from build123d import *

# Parameters (mm, degrees)
SKETCH2_R            = 15.875
BOSS_EXTRUDE1_DEPTH  = 25.4
SKETCH4_R            = 19.05
BOSS_EXTRUDE2_DEPTH  = 25.4
SKETCH5_R            = 22.225
BOSS_EXTRUDE3_DEPTH  = 3.175
SKETCH6_R            = 19.05
BOSS_EXTRUDE4_DEPTH  = 3.175
SKETCH7_R            = 22.225
BOSS_EXTRUDE5_DEPTH  = 43.5102
SKETCH8_R            = 25.4
BOSS_EXTRUDE6_DEPTH  = 77.1398
CUT_EXTRUDE1_DEPTH   = 3.175
SKETCH10_R           = 12.7
BOSS_EXTRUDE7_DEPTH  = 3.175
SKETCH11_R           = 15.875
BOSS_EXTRUDE8_DEPTH  = 3.175
SKETCH12_R           = 12.7
BOSS_EXTRUDE9_DEPTH  = 3.175
SKETCH13_R           = 15.875
BOSS_EXTRUDE10_DEPTH = 3.175


with BuildPart() as part:
    # Sketch2 → Boss-Extrude1 (new body)
    with BuildSketch(Plane.XY):
        Circle(SKETCH2_R)
    extrude(amount=BOSS_EXTRUDE1_DEPTH)

    # Sketch4 → Boss-Extrude2 (add)
    with BuildSketch(Plane.XY.offset(25.4)):
        Circle(SKETCH4_R)
    extrude(amount=BOSS_EXTRUDE2_DEPTH)

    # Sketch5 → Boss-Extrude3 (add)
    with BuildSketch(Plane.XY.offset(50.8)):
        Circle(SKETCH5_R)
    extrude(amount=BOSS_EXTRUDE3_DEPTH)

    # Sketch6 → Boss-Extrude4 (add)
    with BuildSketch(Plane.XY.offset(53.975)):
        Circle(SKETCH6_R)
    extrude(amount=BOSS_EXTRUDE4_DEPTH)

    # Sketch7 → Boss-Extrude5 (add)
    with BuildSketch(Plane.XY.offset(57.15)):
        Circle(SKETCH7_R)
    extrude(amount=BOSS_EXTRUDE5_DEPTH)

    # Sketch8 → Boss-Extrude6 (add)
    with BuildSketch(Plane.XY.offset(100.6602)):
        Circle(SKETCH8_R)
    extrude(amount=BOSS_EXTRUDE6_DEPTH)

    # Sketch9 → Cut-Extrude1 (cut)
    with BuildSketch(Plane(origin=(0, -22.225, 0), x_dir=(-1, 0, 0), z_dir=(0, -1, 0))):
        with BuildLine():
            Line((3.175, -69.3801), (3.175, -88.4301))
            ThreePointArc((3.175, -88.4301), (0, -91.6051), (-3.175, -88.4301))
            Line((-3.175, -88.4301), (-3.175, -69.3801))
            ThreePointArc((-3.175, -69.3801), (0, -66.2051), (3.175, -69.3801))
        make_face()
    extrude(amount=-CUT_EXTRUDE1_DEPTH, mode=Mode.SUBTRACT)

    # Mirror1: part across plane


with BuildPart() as part_1:
    add(part.part)
    add(part.part.mirror(Plane.XY.offset(177.8)))

    # Sketch10 → Boss-Extrude7 (add)
    with BuildSketch(Plane(origin=(0, 0, 0), x_dir=(-1, 0, 0), z_dir=(0, 0, -1))):
        Circle(SKETCH10_R)
    extrude(amount=BOSS_EXTRUDE7_DEPTH)

    # Sketch11 → Boss-Extrude8 (add)
    with BuildSketch(Plane(origin=(0, 0, -3.175), x_dir=(-1, 0, 0), z_dir=(0, 0, -1))):
        Circle(SKETCH11_R)
    extrude(amount=BOSS_EXTRUDE8_DEPTH)

    # Sketch12 → Boss-Extrude9 (add)
    with BuildSketch(Plane.XY.offset(355.6)):
        Circle(SKETCH12_R)
    extrude(amount=BOSS_EXTRUDE9_DEPTH)

    # Sketch13 → Boss-Extrude10 (add)
    with BuildSketch(Plane.XY.offset(358.775)):
        Circle(SKETCH13_R)
    extrude(amount=BOSS_EXTRUDE10_DEPTH)


solid = part_1.part
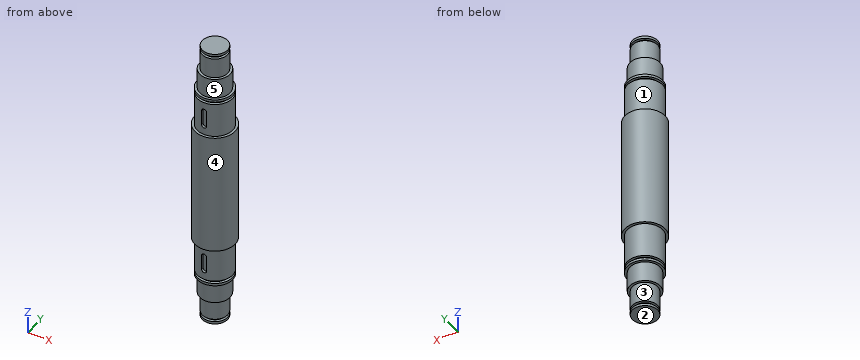
CAD build for the part. Positions are in the model's coordinates, mm. Face numbers are marked on the shaded views. A direction names the side the tool comes from. Give positions to 0.01 mm unless a question says otherwise; leave off trailing zeros. Order: outer loops, then holes, each group sorted by start corner. A loop starts at its lowest first (then second) coordinate and runs counter-clockwise, first axis right, second up. Notation, with made-up numbers: (88.25, 40.5) -> (92.25, 40.5) arc R8 cw to (92.25, 49.5) -> close; hole circle Ø7 at (-25, 77.5). An arc over 180 degrees is marked (long way). Return JSON: item names as keys, results as strings.
Q1. Saw through at A-A (z = 116.5). Write the cut outline in (x, y).
Working result:
{"outline": "circle Ø50.8 at (0, 0)"}
Q2. Which spindle directions (+Z, -Z, +X, -X, +Y, -Y) get a long thin tool onto all of the face, cutting with end or side? Do the marked faces 3, 4 and 5. Say none if no direction does.
Working result:
{"face 3": "-Z", "face 4": "+Z, -Z", "face 5": "+Z"}
Q3. Mould opens along Y. For the marked faces 1 and 2 say: pulls with the +Y half, pulls with the -Y half, needs draft (parallel to the pull), parting line crosses it, or undercut.
Working result:
{"face 1": "parting line crosses it", "face 2": "needs draft"}
Q4. Drill centre lines: line 1 (Z direction, x = 13, y = -3) (3 decimals); line 2 (Z direction, x = 19, y = -10.5) (3 decimals); line 3 (Z direction, x = 4, y = -18). Where is each one in solid material? Low to high.
Working result:
{"line 1": "-6.35 to -3.175, 0 to 355.6, 358.775 to 361.95", "line 2": "50.8 to 53.975, 57.15 to 298.45, 301.625 to 304.8", "line 3": "25.4 to 330.2"}
Q5. Flat gauge pins, fed straight in: pin 1 (10 mm diameter, centred on x = 1, y = 20, fed in from -Z); pin 2 (1.5 mm diameter, centred on y = -20.5, z = 78.5, fed in from +X); pin 3 (0.9 mm diameter, centred on y = -20.5, z = 272.5, fed in from -X); pin 4 (12 mm diameter, centred on x = 8.5, z = 84, fed in from -Y). Where does each tip first touch, or does it go through?
Working result:
{"pin 1": "z = -6.35", "pin 2": "x = 10.19", "pin 3": "x = -9.59", "pin 4": "y = -22"}
